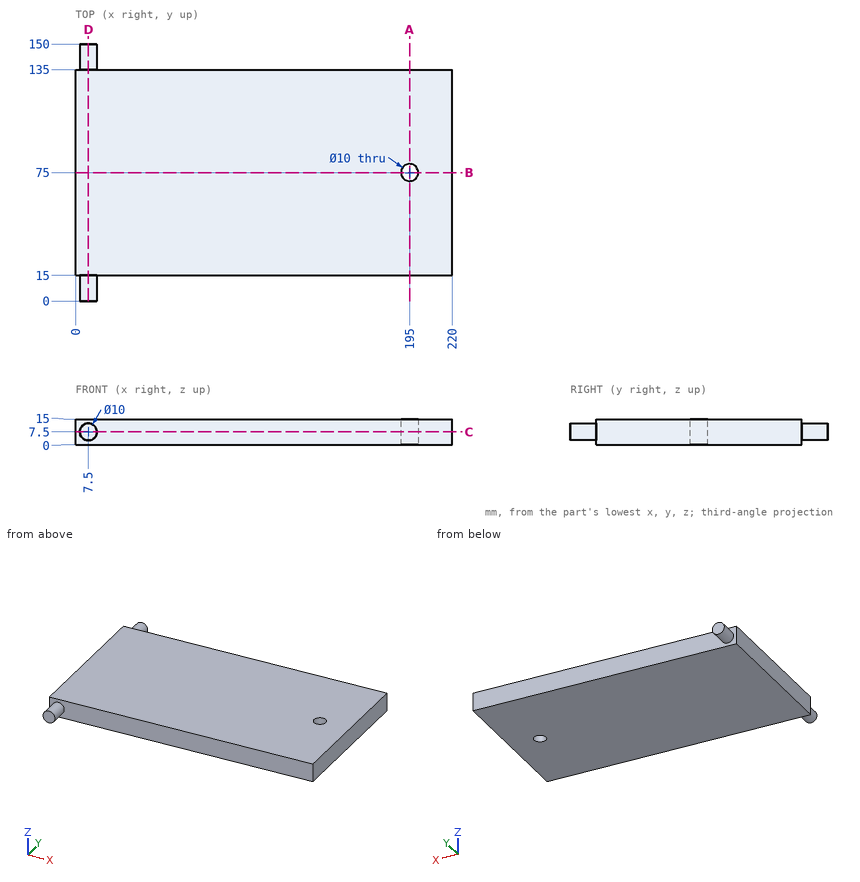
Here's the drawing with two shaded views (mm, measured from the low corner). I have some questions. Give positions to 0.01 mm unless a question says otherwise; leave off trailing zeros. Write each loop counter-clockwise with the first axis right and the second up, starting at its lowest first coordinate (ties: lowest second). Pieces come first, ordered by that corner, then holes. Notation, with made-up numbers: (56, 46) - (70, 46) arc R18 cw to (70, 60) - close; hole circle Ø3 at (-26, 88). An arc over 180 degrees is marked (long way). Write item = value, one per line. Start each with the question number.
1. Imagine slicing it at B-B (y = 75). Please give me the cut outline in (x, z), and give its area (3 significant figures).
2. Imagine slicing it at A-A (x = 195). Please give me the cut outline in (y, z).
3. Imagine slicing it at D-D (x = 7.5). Please give me the cut outline in (y, z), and give its area (3 significant figures).
4. Please list where these lines run through material, in increasing order: line 1 (Y direction, x = 195, z = 4.5); line 2 (Y direction, x = 77.5, z = 13); line 3 (X direction, y = 142, z = 7.5).
5. Imagine slicing it at C-C (z = 7.5). Please give me the cut outline in (x, y), and give its area (3 significant figures).
6. For pin 1 (7.5 mm diameter, centred on x = 143.5, z = 9.5, fed in from +Y); pin 2 (8 mm diameter, centred on x = 195, y = 75, fed in from +Z); pin 3 (4.5 mm diameter, centred on x = 100.5, z = 9.5, fed in from -Y), each with a flat end and sliding along its axis, tell me the tip position at first contact or that it passes through.
Worked answers:
q1.outline = (0, 0) - (190, 0) - (190, 15) - (0, 15) - close; (200, 0) - (220, 0) - (220, 15) - (200, 15) - close
q1.area = 3,150 mm2
q2.outline = (15, 0) - (70, 0) - (70, 15) - (15, 15) - close; (80, 0) - (135, 0) - (135, 15) - (80, 15) - close
q3.outline = (0, 2.5) - (15, 2.5) - (15, 0) - (135, 0) - (135, 2.5) - (150, 2.5) - (150, 12.5) - (135, 12.5) - (135, 15) - (15, 15) - (15, 12.5) - (0, 12.5) - close
q3.area = 2,100 mm2
q4.line_1 = 15 to 70, 80 to 135
q4.line_2 = 15 to 135
q4.line_3 = 2.5 to 12.5
q5.outline = (0, 15) - (2.5, 15) - (2.5, 0) - (12.5, 0) - (12.5, 15) - (220, 15) - (220, 135) - (12.5, 135) - (12.5, 150) - (2.5, 150) - (2.5, 135) - (0, 135) - close; hole circle Ø10 at (195, 75)
q5.area = 26,600 mm2
q6.pin_1 = 135
q6.pin_2 = through
q6.pin_3 = 15
